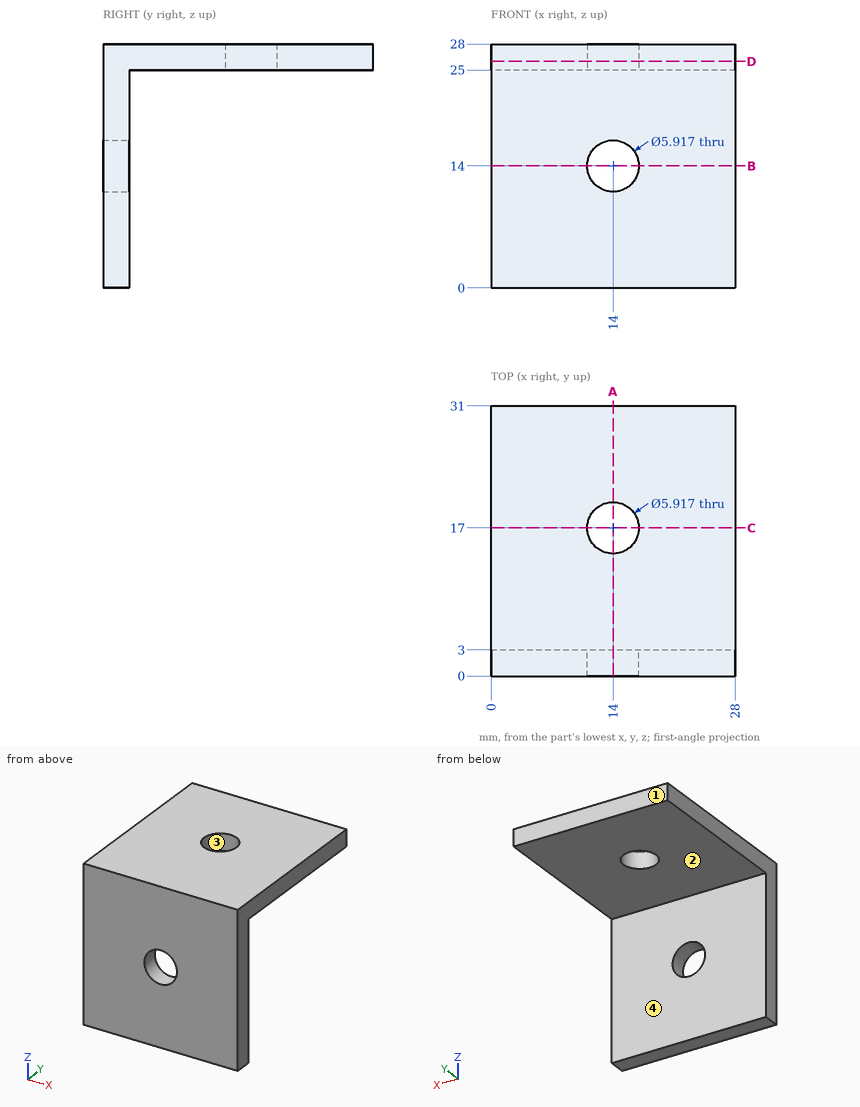
Geometry check sheet. Reference: drawing and pictorial views, mm from the part's lowest x, y, z. A direction names the side the tool comes from. Give positions to 0.01 mm unless a question says otherwise; leave off trailing zeros. Loops run counter-clockwise (first coordinate to the right, second up) from the corner with the lowest first, then second, coordinate; pieces in that order, holes last. Notation, with made-up numbers: (47, -31.75) -> (84, -31.75) arc R18 ccw to (84, -0.75) -> close; hole circle Ø5 at (-36.5, 79). An arc over 180 degrees is marked (long way). Answer in a Markdown table with one row per item. Add a question column.
1) Cross-section at A-A on x = 14. Record the boundary of the cut face in (y, z), and give its area (3 significant figures).
2) Cross-section at B-B on z = 14. Record the boundary of the cut face in (x, y).
3) Gauge pin test, flat ends, axial feed: P1, Ø10, axis at x = 20, z = 13.5, coming from the +Y side; P2, Ø8.5, axis at x = 16, y = 20, coming from the -Z side. Record the tip position at first contact, or that the pin passes through.
4) Cross-section at C-C on y = 17. Record the boundary of the cut face in (x, z).
5) Cross-section at D-D on z = 26. Record the boundary of the cut face in (x, y).
6) Set-up check for the marked faces 1 and 2: record each of +Z, -Z, +X, -X, +Y, -Y from which the full face is reachable in a straight line by a thin tool's end or side.
7) Material ranges on probe 1 along Z at (x, y) = (14, 2.3); probe 2 along Y at (x, z) = (14, 27.3), recorded low to high. Write a range as from..to.
8) Draft check along X on the marked faces 3 and 4. Enter one of: pulls with the +X half, pulls with the -X half, needs draft (parallel to the pull), parting line crosses it, or undercut.
Outcome:
| question | item | result |
|---|---|---|
| 1 | outline | (0, 0) -> (3, 0) -> (3, 11.04) -> (0, 11.04) -> close; (0, 16.96) -> (3, 16.96) -> (3, 25) -> (14.04, 25) -> (14.04, 28) -> (0, 28) -> close; (19.96, 25) -> (31, 25) -> (31, 28) -> (19.96, 28) -> close |
| 1 | area | 132 mm^2 |
| 2 | outline | (0, 0) -> (11.04, 0) -> (11.04, 3) -> (0, 3) -> close; (16.96, 0) -> (28, 0) -> (28, 3) -> (16.96, 3) -> close |
| 3 | P1 | stops at y = 3 |
| 3 | P2 | stops at z = 25 |
| 4 | outline | (0, 25) -> (11.04, 25) -> (11.04, 28) -> (0, 28) -> close; (16.96, 25) -> (28, 25) -> (28, 28) -> (16.96, 28) -> close |
| 5 | outline | (0, 0) -> (28, 0) -> (28, 31) -> (0, 31) -> close; hole circle Ø5.92 at (14, 17) |
| 6 | face 1 | +Z, -Z, +X, -X, +Y |
| 6 | face 2 | -Z, +X, -X, +Y |
| 7 | probe 1 | z = 0..11.04, 16.96..28 |
| 7 | probe 2 | y = 0..14.04, 19.96..31 |
| 8 | face 3 | undercut |
| 8 | face 4 | needs draft |
